Check sheet for the modelled part. Datum: model origin and axes. Units: mm. A direction names the side the tool comes from. Coordinates: 2 decimals unless noted, no trailing zeros. Order: outer loops, then holes, each group sorted by start corner. A loop starts at its lowest first (then second) coordinate and runs counter-clockwise, first axis right, second up. Notation, with made-up numbers: M -34,7 L -17,7 A28 cw -17,45 Z; hole C -6.75,80.25 d10. An arc over 180 degrees is marked long. Answer in a Markdown table with one row per item. Add a question column.
from build123d import *

# Parameters (mm, degrees)
HEX_2_DEPTH = 15


with BuildPart() as part:
    # BodySke → BaseBody (revolve)
    with BuildSketch(Plane.XY, mode=Mode.PRIVATE) as basebody_sk:
        Polygon((0, 0), (0, 10.352), (0.951473244, 12), (40.7, 12), (43.7, 9), (50, 9), (50, 0), align=None)
    revolve(basebody_sk.sketch.rotate(Axis((-12.7, 0, 0), (1, 0, 0)), 90), axis=Axis((-12.7, 0, 0), (1, 0, 0)))

    # Sketch2 → Hex 2 (cut)
    with BuildSketch(Plane.ZY):
        Polygon((3.464101615, 6), (-3.464101615, 6), (-6.92820323, 0), (-3.464101615, -6), (3.464101615, -6), (6.92820323, 0), align=None)
    extrude(amount=-HEX_2_DEPTH, mode=Mode.SUBTRACT)


solid = part.part
1. Go/stop test with flat-tipped pins: pin 1 Ø2 at (x, z) = (41.5, -8) entering from -Y; pin 2 Ø5 at (x, y) = (25.5, -6) entering from -Z; pin 3 Ø5.5 at (x, z) = (4, 1.5) entering from +Y; pin 4 Ø1.5 at (x, z) = (35, 5) entering from +Y. Record where each tip stops, or that it passes through.
2. Scan lines: line 1 (X direction, y = 3.25, z = 4); line 2 (Y direction, x = 9.5, z = 3.5); line 3 (Y direction, x = 2, z = 6.75). Record each from-to range of solid material in increasing order.
3. Set-up check for faces 5 (the cylindrical face through (21.104, -3.604, 11.446)), 6 (the flat face through (7, 6, 0)): record each of +Z, -Z, +X, -X, +Y, -Y from which the full face is reachable in a straight line by a thin tool's end or side.
4. Section check B-B on x = 30.5. Enter the section's corners in (y, z), then the cut area to 3 significant figures.
5. Release check for a two-part mould opening along Z. For faces 1 (the flat face through (7.395, -3.042, 5.172)), 2 (the flat face through (0, 4, 5)), 3 (the cylindrical face through (46.894, -6.083, -6.633)), 4 (the flat face through (7.4, -2.96, -5.22)) record: released by +Z, released by -Z, zero draft, split by the parting line, or undercut.
6. Section check A-A on z = 0. Enter the section's corners in (x, y), then the cut area to 3 significant figures.
Result sheet:
| question | item | result |
|---|---|---|
| 1 | pin 1 | y = -9.45 |
| 1 | pin 2 | z = -11.48 |
| 1 | pin 3 | y = 12 |
| 1 | pin 4 | y = 11.22 |
| 2 | line 1 | 15 to 50 |
| 2 | line 2 | -11.48 to -5.94, 5.94 to 11.48 |
| 2 | line 3 | -9.92 to -0.31, 0.31 to 9.92 |
| 3 | face 5 | +X, -X |
| 3 | face 6 | -X |
| 4 | outline | C 0,0 d24 |
| 4 | area | 452 mm^2 |
| 5 | face 1 | undercut |
| 5 | face 2 | zero draft |
| 5 | face 3 | split by the parting line |
| 5 | face 4 | undercut |
| 6 | outline | M 0,-10.35 L 0.95,-12 L 40.7,-12 L 43.7,-9 L 50,-9 L 50,9 L 43.7,9 L 40.7,12 L 0.95,12 L 0,10.35 L 0,6 L 15,6 L 15,-6 L 0,-6 Z |
| 6 | area | 972 mm^2 |
